Verification items for the finished model (mm, model axes). A direction names the side the tool comes from. Round coordinates to 2 decimals unless told otherwise and drop trailing zeros. Order: outer loops, then holes, each group sorted by start corner. A loop starts at its lowest first (then second) coordinate and runs counter-clockwise, first axis right, second up. Notation, with made-up numbers: M 88.5,35.25 L 146.5,35.25 A3 ccw 146.5,40.25 Z; hole C -30.5,-1.75 d4. An arc over 180 degrees is marked long. Use one line per item in the form item = value. Start each with the question number.
Item 1: Cross-section at B-B on x = 129. Enter the section's corners in (y, z), then the cut area to 3 significant figures.
Item 2: Go/stop test with flat-tipped pins: pin 1 Ø5 at (x, z) = (155, 45) entering from +Y; pin 2 Ø8 at (x, y) = (147.5, -104) entering from -Z. Record where each tip stops, or that it passes through.
Item 3: Tool access check on faces 1 (the flat face through (88, -81, 0)), 2 (the cylindrical face through (160.255, 12.522, 70.967)). Record the directions out of +Z, -Z, +X, -X, +Y, -Y that give a thin tool (end or side, any length) a straight path to the whole face; none if there is none.
Item 4: Cross-section at A-A on z = 8.5. Enter the section's corners in (x, y).
Item 5: Thickness scan on probe 1 along Y at (x, z) = (163, 11); probe 2 along X at (y, z) = (9, 68). Record the ranges inside material, lowest first. Write a range as [from, to].
from build123d import *

# Parameters (mm, degrees)
F0_W     = 177.8
F0_H     = 165.1
F1_DEPTH = 76.2
F2_R     = 6.35
F3_DEPTH = 25.4


with BuildPart() as f1:
    # F0 (on Top) → F1 (new body)
    with BuildSketch(Plane.XY):
        with Locations((88.9, -82.55)):
            Rectangle(F0_W, F0_H)
    extrude(amount=F1_DEPTH)

    # F2 (on face) → F3 (join)
    with BuildSketch(Plane(origin=(0, 0, 0), x_dir=(-1, 0, 0), z_dir=(0, 1, 0))):
        with Locations((-155.575, 66.675)):
            Circle(F2_R)
        with Locations((-22.225, 66.675)):
            Circle(F2_R)
    extrude(amount=F3_DEPTH)


solid = f1.part
Output values:
q1.outline = M -165.1,0 L 0,0 L 0,76.2 L -165.1,76.2 Z
q1.area = 12,600 mm2
q2.pin_1 = 0
q2.pin_2 = 0
q3.face_1 = -Z, +X, -X, +Y, -Y
q3.face_2 = +Y
q4.outline = M 0,-165.1 L 177.8,-165.1 L 177.8,0 L 0,0 Z
q5.probe_1 = [-165.1, 0]
q5.probe_2 = [16.01, 28.44], [149.36, 161.79]
